from build123d import *

# Parameters (mm, degrees)
F0_R           = 15.875
F1_DEPTH       = 152.4
F3_DEPTH       = 127
F4_R           = 3.175
F5_DEPTH       = 152.4
F8_DEPTH       = 101.6
F10_DEPTH      = 25.401
F10_DEPTH_BACK = 127.001
F12_DEPTH      = 152.401
F13_W          = 19.05
F13_H          = 22.86
F14_DEPTH      = 15.876
F14_DEPTH_BACK = 15.876


with BuildPart() as f1:
    # F0 (on Top) → F1 (new body)
    with BuildSketch(Plane.XY):
        Circle(F0_R)
    extrude(amount=F1_DEPTH)

    # F2 (on face) → F3 (cut)
    with BuildSketch(Plane.XY.offset(152.4)):
        Polygon((4.6622561211, 4.6622561211), (-4.318, -4.318), (4.6622561211, -13.2982561211), (13.6425122421, -4.318), align=None)
    extrude(amount=-F3_DEPTH, mode=Mode.SUBTRACT)

    # F4 (on face) → F5 (cut)
    with BuildSketch(Plane.XY.offset(152.4)):
        with Locations((4.6622561211, -4.318)):
            Circle(F4_R)
    extrude(amount=-F5_DEPTH, mode=Mode.SUBTRACT)

    # F7 (on offset) → F8 (cut)
    with BuildSketch(Plane.XY.offset(127)):
        Polygon((8.9802561211, -8.9802561211), (0, 0), (-17.9605122421, -17.9605122421), (-8.9802561211, -26.9407683632), align=None)
    extrude(amount=-F8_DEPTH, mode=Mode.SUBTRACT)

    # F9 (on face) → F10 (cut, two sides)
    with BuildSketch(Plane.XY.offset(25.4)) as f10_sk:
        Polygon((-6.8689398237, -19.4412983932), (5.1112689271, -7.4610896424), (1.5191664787, -3.8689871939), (-10.4610422721, -15.8491959447), align=None)
    extrude(amount=-F10_DEPTH, mode=Mode.SUBTRACT)
    extrude(f10_sk.sketch, amount=F10_DEPTH_BACK, mode=Mode.SUBTRACT)

    # F11 (on face) → F12 (cut, through all)
    with BuildSketch(Plane.XY.offset(152.4)):
        Polygon((-23.2781873974, 10.1192935667), (-26.9931931626, 10.1192935667), (-26.9931931626, -0.6757064333), (-7.9431931626, -0.6757064333), (-5.7593395008, 0), (-5.7593395008, 4.2418), align=None)
    extrude(amount=-F12_DEPTH, mode=Mode.SUBTRACT)

    # F13 (on Front) → F14 (cut, two sides)
    with BuildSketch(Plane.XZ) as f14_sk:
        with Locations((-15.875, 76.2)):
            Rectangle(F13_W, F13_H)
    extrude(amount=-F14_DEPTH, mode=Mode.SUBTRACT)
    extrude(f14_sk.sketch, amount=F14_DEPTH_BACK, mode=Mode.SUBTRACT)


solid = f1.part
The listing builds one solid part. Answer for the finished solid, in the listing's coordinates (mm). A direction names the side the tool comes from. Round coordinates to 2 decimals unless told otherwise and drop trailing zeros. Write each loop counter-clockwise with the first axis right and the second up, starting at its lowest first coordinate (ties: lowest second). Pieces come first, ordered by that corner, then holes. Notation, with made-up numbers: M 85.25,-15 L 125.25,-15 A13 cw 125.25,-10 Z; hole C 57,2.25 d3. An arc over 180 degrees is marked long. Write each question's results on one line, items separated by ' | '. Start each with the question number.
Item 1: A cutting plane is placed at D-D on z = 10.5. Write down the section's boundary in (x, y) (3 decimals).
Item 2: A cutting plane is placed at A-A on z = 43. Write down the section's boundary in (x, y) (3 decimals).
Item 3: A cutting plane is placed at B-B on y = 12. Write down the section's boundary in (x, z).
Item 4: For faces 5 (the face through (-12, -0.676, 120)), 6 (the face through (9.215, 0.109, 89.789)), 7 (the face through (1, -4, 25.4)), 8 (the face through (-11, -4, 87.63)), 9 (the face through (-3.27, -8.66, 12.88)), determine the directions among +Z, -Z, +X, -X, +Y, -Y from which every point of the face is accessible in a straight line to the end or side of a thin tool.
Item 5: For a pull along X with two mould halves and no side action, classify faces 1 (the face through (-9, 9, 87.63)), 2 (the face through (-6, -9, 127)), 3 (the face through (3.296, -11.932, 139.878)), 4 (the face through (-6.35, 9, 76)) as pulls with the +X half, pulls with the -X half, needs draft (parallel to the pull), parting line crosses it, or undercut.
Item 6: A cutting plane is placed at C-C on x = 0. Write down the section's boundary in (y, z) (3 decimals).
Item 7: Straight lines are drawn through the part: L1, parallel to Z at x = -12, y = -3; L2, parallel to Y at x = -11, z = 46; L3, parallel to X at y = -1, z = 22.5. For each, find the intervals that lie inside material, in ascending order. Write a range as [from, to].
Item 8: Flat-ended cylindrical pins translate along their axes: pin 1 Ø5 at (x, z) = (3, 64.5) entering from -Y; pin 2 Ø3 at (y, z) = (10.5, 74) entering from -X; pin 3 Ø2.5 at (x, y) = (-9, 7) entering from -Z; pin 4 Ø6 at (x, y) = (1, -4) entering from +Z. Find the tip coordinate at first contact, or state that the pin passes through.
Check sheet entries:
1) outline: M -15.861,-0.676 A15.875 ccw -8.203,-13.591 L 1.519,-3.869 A3.175 cw long 5.111,-7.461 L -3.014,-15.586 A15.875 ccw long -14.21,7.077 L -5.759,4.242 L -5.759,0 L -7.943,-0.676 Z
2) outline: M -15.861,-0.676 A15.875 ccw -11.225,-11.225 L 4.662,4.662 L 13.643,-4.318 L 2.245,-15.715 A15.875 ccw long -14.21,7.077 L -5.759,4.242 L -5.759,0 L -7.943,-0.676 Z
3) outline: M -10.39,0 L 10.39,0 L 10.39,152.4 L -10.39,152.4 L -10.39,87.63 L -6.35,87.63 L -6.35,64.77 L -10.39,64.77 Z
4) face 5: +Z, -Z, -X | face 6: +Z | face 7: none | face 8: -X, +Y, -Y | face 9: +Z, -Z
5) face 1: needs draft | face 2: undercut | face 3: undercut | face 4: pulls with the -X half
6) outline: M -15.875,0 L -12.572,0 L -12.572,25.4 L -15.875,25.4 Z; M -15.875,127 L -12.572,127 L -12.572,152.4 L -15.875,152.4 Z; M -5.388,0 L 15.875,0 L 15.875,152.4 L 0,152.4 L 0,25.4 L -5.388,25.4 Z
7) L1: [0, 64.77], [87.63, 152.4] | L2: [-11, -0.68], [6, 11.45] | L3: [-15.84, 15.84]
8) pin 1: y = -15.72 | pin 2: x = -6.35 | pin 3: z = 0 | pin 4: z = 25.4
